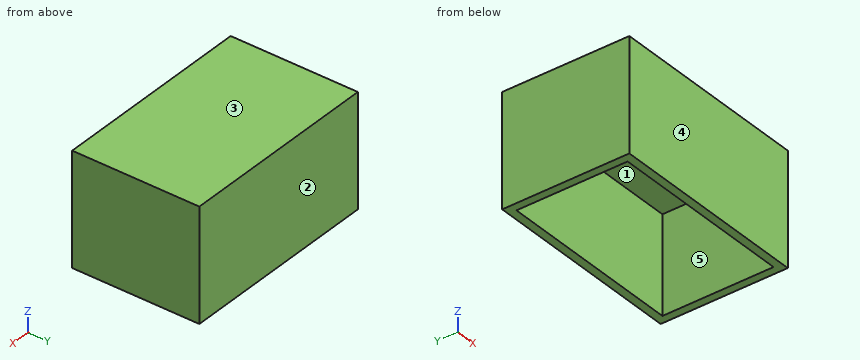
from build123d import *

# Parameters (mm, degrees)
F0_W     = 20.13
F0_H     = 12.6
F1_DEPTH = 11.11
F2_W     = 18.54
F2_H     = 11.01
F3_DEPTH = 9.62


with BuildPart() as f1:
    # F0 (on Top) → F1 (new body)
    with BuildSketch(Plane.XY):
        Rectangle(F0_W, F0_H)
    extrude(amount=-F1_DEPTH)

    # F2 (on face) → F3 (cut)
    with BuildSketch(Plane(origin=(0, 0, -11.11), x_dir=(1, 0, 0), z_dir=(0, 0, -1))):
        Rectangle(F2_W, F2_H)
    extrude(amount=-F3_DEPTH, mode=Mode.SUBTRACT)


solid = f1.part
Check sheet for the modelled part. Datum: model origin and axes. Units: mm. Face numbers are marked on the shaded views. A direction names the side the tool comes from. Round coordinates to 2 decimals unless told otherwise and drop trailing zeros. Write each loop counter-clockwise with the first axis right and the second up, starting at its lowest first coordinate (ties: lowest second). Pieces come first, ordered by that corner, then holes. Notation, with made-up numbers: (-21.75, 68) -> (11.25, 68) arc R12 cw to (11.25, 88) -> close; hole circle Ø3 at (-19, 48.5). An arc over 180 degrees is marked (long way). Answer as CSV lines item,"result". Start each with the question number.
1) Release check for a two-part mould opening along Y. For the marked faces 3, 4 and 5 record: pulls with the +Y half, pulls with the -Y half, needs draft (parallel to the pull), parting line crosses it, or undercut.
2) Go/stop test with a flat-tipped pin: P1, Ø5.5, axis at x = 1, y = -0.5, coming from the -Z side. Record where the tip stops, or that it passes through.
3) Section check A-A on z = -10.25. Enter the section's corners in (x, y) (3 decimals), and give its area (3 significant figures).
4) Section check B-B on y = 3.25. Enter the section's corners in (x, z) (3 decimals).
5) Tool access check on the marked faces 1 and 2. Record the directions out of +Z, -Z, +X, -X, +Y, -Y that give a thin tool (end or side, any length) a straight path to the whole face; none if there is none.
6) Material ranges on line 1 (X direction, y = -2.5, z = -5.75) (3 decimals); line 2 (Y direction, x = 6, z = -6) (3 decimals); line 3 (Z direction, x = 7.75, y = -1), recorded low to high. Write a range as from..to.
7) Section check C-C on x = -7.25. Enter the section's corners in (y, z) (3 decimals).
Found:
1,face 3,"needs draft"
1,face 4,"pulls with the -Y half"
1,face 5,"undercut"
2,P1,"stops at z = -1.49"
3,outline,"(-10.065, -6.3) -> (10.065, -6.3) -> (10.065, 6.3) -> (-10.065, 6.3) -> close; hole (-9.27, -5.505) -> (9.27, -5.505) -> (9.27, 5.505) -> (-9.27, 5.505) -> close"
3,area,"49.5 mm^2"
4,outline,"(-10.065, -11.11) -> (-9.27, -11.11) -> (-9.27, -1.49) -> (9.27, -1.49) -> (9.27, -11.11) -> (10.065, -11.11) -> (10.065, 0) -> (-10.065, 0) -> close"
5,face 1,"-Z"
5,face 2,"+Z, -Z, +X, -X, +Y"
6,line 1,"x = -10.065..-9.27, 9.27..10.065"
6,line 2,"y = -6.3..-5.505, 5.505..6.3"
6,line 3,"z = -1.49..0"
7,outline,"(-6.3, -11.11) -> (-5.505, -11.11) -> (-5.505, -1.49) -> (5.505, -1.49) -> (5.505, -11.11) -> (6.3, -11.11) -> (6.3, 0) -> (-6.3, 0) -> close"
